```python
from build123d import *

# Parameters (mm, degrees)
SALIENTE_EXTRUIR1_DEPTH   = 6
SALIENTE_EXTRUIR1_2_DEPTH = 6
SALIENTE_EXTRUIR2_REACH   = 84.292
CROQUIS2_R                = 3


with BuildPart() as part:
    # Croquis1 → Saliente-Extruir1 (new body)
    with BuildSketch(Plane(origin=(0, 0, 0), x_dir=(0, 0, -1), z_dir=(1, 0, 0))):
        Polygon((56, 0), (62, 0), (62, 60), (56, 60), (56, 54), align=None)
    extrude(amount=SALIENTE_EXTRUIR1_DEPTH)


with BuildPart() as body_2:
    # Croquis1 → Saliente-Extruir1 2 (new body)
    with BuildSketch(Plane(origin=(0, 0, 0), x_dir=(0, 0, -1), z_dir=(1, 0, 0))):
        Polygon((0, 0), (6, 0), (6, 54), (6, 60), (0, 60), align=None)
    extrude(amount=SALIENTE_EXTRUIR1_2_DEPTH)

    # Croquis2 → Saliente-Extruir2 (add, up to next)
    with BuildSketch(Plane.XY.offset(-56), mode=Mode.PRIVATE) as saliente_extruir2_sk1:
        with Locations(Location((3, 57, 0), (0, 0, 180))):
            Circle(CROQUIS2_R)
    saliente_extruir2_tool1 = extrude(saliente_extruir2_sk1.sketch, amount=SALIENTE_EXTRUIR2_REACH, mode=Mode.PRIVATE) - body_2.part

    add(part.part)  # Saliente-Extruir2 merges part
    add(saliente_extruir2_tool1.solids().sort_by_distance((3, 57, -56))[0])


solid = body_2.part
```
Part model, mm, in its own coordinate system. A direction names the side the tool comes from. Coordinates: 2 decimals unless noted, no trailing zeros. Order: outer loops, then holes, each group sorted by start corner. A loop starts at its lowest first (then second) coordinate and runs counter-clockwise, first axis right, second up. Notation, with made-up numbers: (33.25, 45) -> (83.25, 45) arc R21 ccw to (83.25, 63) -> close; hole circle Ø9 at (0, 57). An arc over 180 degrees is marked (long way). Put each result on its own line as item: value. Start each with the question number.
(1) Which spindle directions (+Z, -Z, +X, -X, +Y, -Y) get a long thin tool onto all of the face, cutting with end or side? Do faces 5 (the face through (0.7, 59.4, -56)), 6 (the face through (3, 54, -31)), 7 (the face through (5.4, 59.4, -6)). Say none if no direction does.
(2) Probe line 1 along Z through (x, y) = (4.25, 3); line 2 along Y through (x, z) = (3.1, -39.5); line 3 along Y through (x, z) = (5.7, -24.5). List the from-to ranges inside material, lowest first. Write a range as [from, to].
(3) Band-saw the part on D-D (x = 1). Give the cut face in (y, z), then the cut area to 3 significant figures.
(4) Band-saw the part on A-A (y = 30). Give the cut face in (x, z), then the cut area to 3 significant figures.
(5) Band-saw the part on C-C (z = -48). Give the cut face in (x, y), then the cut area to 3 significant figures.
(6) Mould opens along Z. For faces 1 (the face through (3, 30, 0)), 2 (the face through (3, 60, -3)), 3 (the face through (3, 29, -56)), 4 (the face through (0.6, 59.3, -6)) say: pulls with the +Z half, pulls with the -Z half, needs draft (parallel to the pull), parting line crosses it, or undercut.
(7) Band-saw the part on B-B (x = 4.2). Give the cut face in (y, z).
Determined:
1. face 5: -X, +Y
1. face 6: none
1. face 7: +X, +Y
2. line 1: z = [-62, -56], [-6, 0]
2. line 2: y = [54, 60]
2. line 3: y = [55.69, 58.31]
3. outline: (0, -62) -> (60, -62) -> (60, -56) -> (59.24, -56) -> (59.24, -6) -> (60, -6) -> (60, 0) -> (0, 0) -> (0, -6) -> (54.76, -6) -> (54.76, -56) -> (0, -56) -> close
3. area: 944 mm²
4. outline: (0, -62) -> (6, -62) -> (6, -56) -> (0, -56) -> close; (0, -6) -> (6, -6) -> (6, 0) -> (0, 0) -> close
4. area: 72.0 mm²
5. outline: circle Ø6 at (3, 57)
5. area: 28.3 mm²
6. face 1: pulls with the +Z half
6. face 2: needs draft
6. face 3: undercut
6. face 4: undercut
7. outline: (0, -62) -> (60, -62) -> (60, -56) -> (59.75, -56) -> (59.75, -6) -> (60, -6) -> (60, 0) -> (0, 0) -> (0, -6) -> (54.25, -6) -> (54.25, -56) -> (0, -56) -> close
